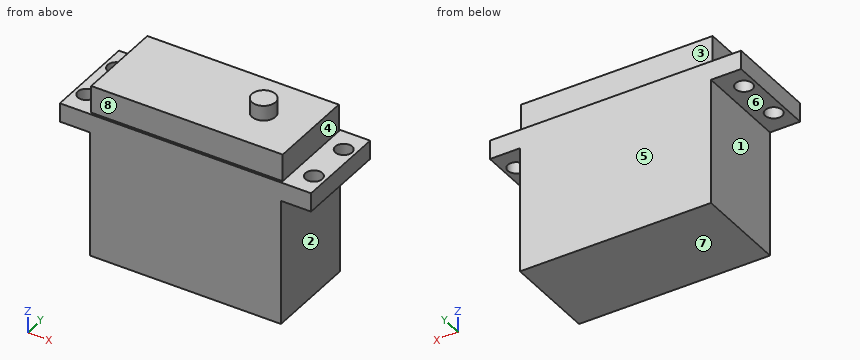
from build123d import *

# Parameters (mm, degrees)
SKETCH1_W            = 40.6
SKETCH1_H            = 19.8
BOSS_EXTRUDE1_DEPTH  = 26.8
SKETCH2_W            = 53.4
SKETCH2_H            = 19.8
BOSS_EXTRUDE2_DEPTH  = 4
M3_CLEARANCE_HOLE1_D = 3.6
SKETCH6_W            = 40.7
SKETCH6_H            = 18.8
BOSS_EXTRUDE3_DEPTH  = 5.8
SKETCH7_R            = 2.5
BOSS_EXTRUDE4_DEPTH  = 3.2


with BuildPart() as part:
    # Sketch1 → Boss-Extrude1 (new body)
    with BuildSketch(Plane.XY):
        with Locations((20.3, 9.9)):
            Rectangle(SKETCH1_W, SKETCH1_H)
    extrude(amount=BOSS_EXTRUDE1_DEPTH)

    # Sketch2 → Boss-Extrude2 (add)
    with BuildSketch(Plane.XY.offset(26.8)):
        with Locations((20.3, 9.9)):
            Rectangle(SKETCH2_W, SKETCH2_H)
    extrude(amount=BOSS_EXTRUDE2_DEPTH)

    # M3 Clearance Hole1 (through all)
    with Locations(Plane.XY.offset(30.8)):
        with Locations((-3.9, 14.9), (-3.9, 4.9), (44.5, 4.9), (44.5, 14.9)):
            Hole(M3_CLEARANCE_HOLE1_D / 2)

    # Sketch6 → Boss-Extrude3 (add)
    with BuildSketch(Plane.XY.offset(30.8)):
        with Locations((20.3, 9.9)):
            Rectangle(SKETCH6_W, SKETCH6_H)
    extrude(amount=BOSS_EXTRUDE3_DEPTH)

    # Sketch7 → Boss-Extrude4 (add)
    with BuildSketch(Plane.XY.offset(36.6)):
        with Locations(Location((30.65, 9.9, 0), (0, 0, 180))):
            Circle(SKETCH7_R)
    extrude(amount=BOSS_EXTRUDE4_DEPTH)


solid = part.part
Model file for the job. Use its own axes, mm. Face numbers are marked on the shaded views. A direction names the side the tool comes from. Round coordinates to 2 decimals unless told otherwise and drop trailing zeros. Loops run counter-clockwise (first coordinate to the right, second up) from the corner with the lowest first, then second, coordinate; pieces in that order, holes last.
1. Band-saw the part on A-A, the plane y = 14.9. List the corners of the cut face in (x, z).
Check values:
outline: (-6.4, 26.8) - (-5.7, 26.8) - (-5.7, 30.8) - (-6.4, 30.8) - close; (-2.1, 26.8) - (0, 26.8) - (0, 0) - (40.6, 0) - (40.6, 26.8) - (42.7, 26.8) - (42.7, 30.8) - (40.65, 30.8) - (40.65, 36.6) - (-0.05, 36.6) - (-0.05, 30.8) - (-2.1, 30.8) - close; (46.3, 26.8) - (47, 26.8) - (47, 30.8) - (46.3, 30.8) - close
2. Wall check: probe 1 along Y at (x, z) = (44.5, 29.5); probe 2 along X at (y, z) = (7.5, 35); probe 3 along Z at (x, y) = (32, 5.75). Give the ranges that are in metal, low to high.
Check values:
probe 1: y = 0 to 3.1, 6.7 to 13.1, 16.7 to 19.8
probe 2: x = -0.05 to 40.65
probe 3: z = 0 to 36.6
3. Band-saw the part on D-D, the plane y = 4.25. List the corners of the cut face in (x, z).
Check values:
outline: (-6.4, 26.8) - (-5.58, 26.8) - (-5.58, 30.8) - (-6.4, 30.8) - close; (-2.22, 26.8) - (0, 26.8) - (0, 0) - (40.6, 0) - (40.6, 26.8) - (42.82, 26.8) - (42.82, 30.8) - (40.65, 30.8) - (40.65, 36.6) - (-0.05, 36.6) - (-0.05, 30.8) - (-2.22, 30.8) - close; (46.18, 26.8) - (47, 26.8) - (47, 30.8) - (46.18, 30.8) - close
4. Band-saw the part on B-B, the plane x = -3.9. List the corners of the cut face in (y, z), and give its area (3 significant figures).
Check values:
outline: (0, 26.8) - (3.1, 26.8) - (3.1, 30.8) - (0, 30.8) - close; (6.7, 26.8) - (13.1, 26.8) - (13.1, 30.8) - (6.7, 30.8) - close; (16.7, 26.8) - (19.8, 26.8) - (19.8, 30.8) - (16.7, 30.8) - close
area: 50.4 mm2
5. Drop flat-ended pins along their axis: P1, Ø4.5, axis at x = 23.5, z = 34, coming from the +Y side; P2, Ø4, axis at x = 9.5, y = 4.5, coming from the -Z side; P3, Ø1.7, axis at x = 18, z = 35, coming from the -Y side; P4, Ø3, axis at x = -4.5, y = 10.5, coming from the -Z side. Give the stop position or say it passes through.
Check values:
P1: stops at y = 19.3
P2: stops at z = 0
P3: stops at y = 0.5
P4: stops at z = 26.8
6. Mould opens along X. For the marked faces 1, 2 and 3 say: +X half, -X half, draft (parallel to the pull), parting line (faces both ways), or undercut.
Check values:
face 1: -X half
face 2: +X half
face 3: draft
7. Tool access for the marked faces 4, 5, 6, 7 and 8: list every direction of +Z, -Z, +X, -X, +Y, -Y with a clear straight run to the whole face (end or side of a thin tool).
Check values:
face 4: +Z, +X, +Y, -Y
face 5: +Z, -Z, +X, -X, +Y
face 6: -Z, -X, +Y, -Y
face 7: -Z, +X, -X, +Y, -Y
face 8: +Z, +X, -X, -Y
8. Band-saw the part on C-C, the plane x = 29. List the corners of the cut face in (y, z), and give its area (3 significant figures).
Check values:
outline: (0, 0) - (19.8, 0) - (19.8, 30.8) - (19.3, 30.8) - (19.3, 36.6) - (11.78, 36.6) - (11.78, 39.8) - (8.02, 39.8) - (8.02, 36.6) - (0.5, 36.6) - (0.5, 30.8) - (0, 30.8) - close
area: 731 mm2
